For this review, use the dimensioned drawing (mm, ordinates from the lowest corner) and the shaded views. A direction names the side the tool comes from. Coordinates: 2 decimals unless noted, no trailing zeros. Order: outer loops, then holes, each group sorted by start corner. A loop starts at its lowest first (then second) coordinate and runs counter-clockwise, first axis right, second up. Notation, with made-up numbers: (-10, 5.25) -> (8, 5.25) arc R14 cw to (8, 17.25) -> close; hole circle Ø7 at (-29.5, 9). An arc over 180 degrees is marked (long way). Return JSON: item names as keys, results as strings. Group by question number.
Item 1: Insertion check: pin 1 (3 mm diameter, centred on x = 33, y = 21.5, fed in from +Z); pin 2 (2.5 mm diameter, centred on y = 1.5, z = 9.5, fed in from -X); pin 3 (4 mm diameter, centred on y = 10.5, z = 9, fed in from +X); pin 4 (14.5 mm diameter, centred on x = 41.35, y = 32, fed in from -Z). Each pin has a flat end and moves straight along its axis. Give the tip position at first contact, or say it passes through.
Item 2: Machinability: for the marked faces 1, 2 and 3, which of the approach directions +Z, -Z, +X, -X, +Y, -Y give a long, thin tool a straight path to every point of the face, cutting with its end or side? Answer none if there is none.
Item 3: Take a section at C-C (z = 11). Write out the cut boundary in (x, y).
Item 4: Take a section at B-B (x = 37). Write out the cut boundary in (y, z), then the cut area to 3 significant figures.
Item 5: Take a section at D-D (y = 26). Write out the cut boundary in (x, z), then the cut area to 3 significant figures.
Item 6: For line 1 along Y through (x, z) = (14.65, 9.3); line 2 along Y through (x, z) = (22, 3.25); line 3 along X through (y, z) = (11.5, 11.5), list the stretches that pass through material, from the lowest coordinate up.
Item 7: Draft analysis for pull direction Y (two halves, no side actions). For the marked faces 4, 5 and 6, state which applies: +Y half, -Y half, draft (parallel to the pull), parting line (faces both ways), or undercut.
Item 8: Take a section at A-A (y = 32). Write out the cut boundary in (x, z).
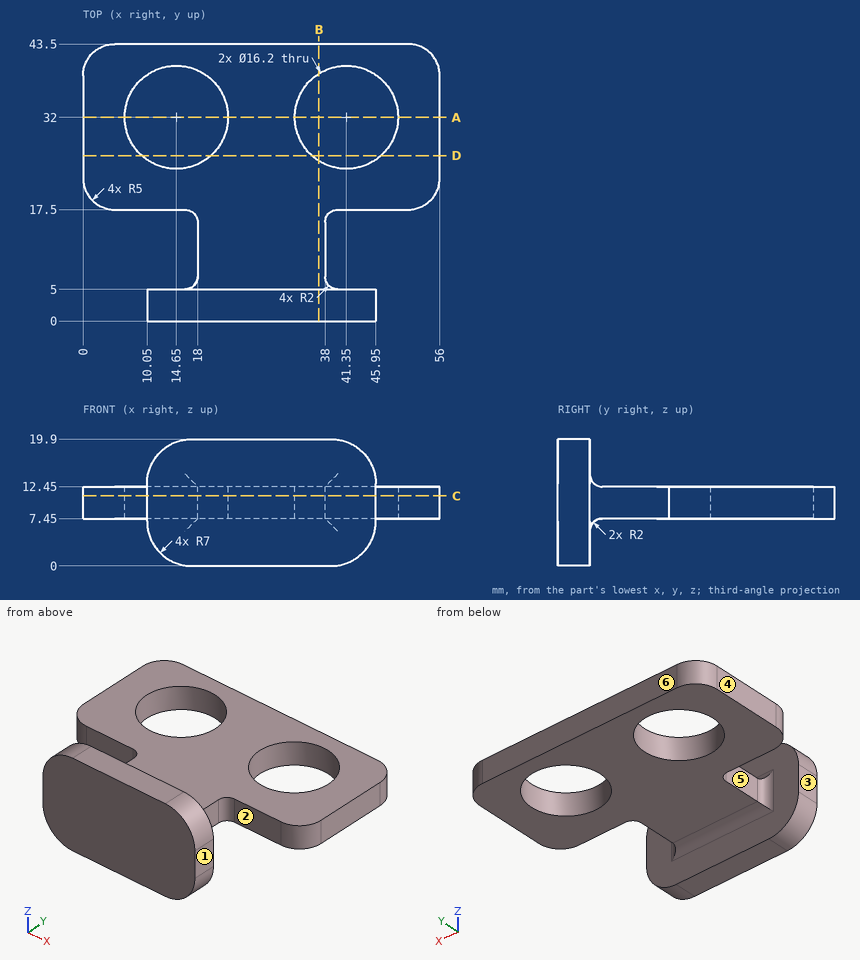
Findings below:
{
 "1": {"pin 1": "stops at z = 12.45", "pin 2": "stops at x = 10.05", "pin 3": "stops at x = 38", "pin 4": "passes through"},
 "2": {"face 1": "+Z, -Z, +X, -Y", "face 2": "+Z, -Z, +X", "face 3": "+Z, -Z, -X, -Y"},
 "3": {"outline": "(0, 22.5) arc R5 ccw to (5, 17.5) -> (16, 17.5) arc R2 cw to (18, 15.5) -> (18, 7) arc R2 cw to (16, 5) -> (10.05, 5) -> (10.05, 0) -> (45.95, 0) -> (45.95, 5) -> (40, 5) arc R2 cw to (38, 7) -> (38, 15.5) arc R2 cw to (40, 17.5) -> (51, 17.5) arc R5 ccw to (56, 22.5) -> (56, 38.5) arc R5 ccw to (51, 43.5) -> (5, 43.5) arc R5 ccw to (0, 38.5) -> close; hole circle Ø16.2 at (14.65, 32); hole circle Ø16.2 at (41.35, 32)"},
 "4": {"outline": "(0, 0) -> (5, 0) -> (5, 5.45) arc R2 cw to (7, 7.45) -> (25.17, 7.45) -> (25.17, 12.45) -> (7, 12.45) arc R2 cw to (5, 14.45) -> (5, 19.9) -> (0, 19.9) -> close; (38.83, 7.45) -> (43.5, 7.45) -> (43.5, 12.45) -> (38.83, 12.45) -> close", "area": "225 mm2"},
 "5": {"outline": "(0, 7.45) -> (9.21, 7.45) -> (9.21, 12.45) -> (0, 12.45) -> close; (20.09, 7.45) -> (35.91, 7.45) -> (35.91, 12.45) -> (20.09, 12.45) -> close; (46.79, 7.45) -> (56, 7.45) -> (56, 12.45) -> (46.79, 12.45) -> close", "area": "171 mm2"},
 "6": {"line 1": "y = 0 to 5, 17.5 to 23.9, 40.1 to 43.5", "line 2": "y = 0 to 5", "line 3": "x = 18 to 38"},
 "7": {"face 4": "draft", "face 5": "undercut", "face 6": "+Y half"},
 "8": {"outline": "(0, 7.45) -> (6.55, 7.45) -> (6.55, 12.45) -> (0, 12.45) -> close; (22.75, 7.45) -> (33.25, 7.45) -> (33.25, 12.45) -> (22.75, 12.45) -> close; (49.45, 7.45) -> (56, 7.45) -> (56, 12.45) -> (49.45, 12.45) -> close"}
}
